```python
from build123d import *

# Parameters (mm, degrees)
F3_DEPTH = 10


with BuildPart() as f3:
    # F2 (on face) → F3 (new body)
    with BuildSketch(Plane.XY):
        with BuildLine():
            ThreePointArc((-207.1709679964, -147.5133103132), (-207.6520447758, -144.8452854186), (-209.0346813202, -142.5133103132))
            Line((-209.0346813202, -142.5133103132), (-209.0346813202, -152.5133103132))
            ThreePointArc((-209.0346813202, -152.5133103132), (-207.6520447758, -150.1813352079), (-207.1709679964, -147.5133103132))
        make_face()
        with BuildLine():
            Line((-139.082004335, -142.5133103132), (-209.0346813202, -142.5133103132))
            ThreePointArc((-209.0346813202, -142.5133103132), (-207.6520447758, -144.8452854186), (-207.1709679964, -147.5133103132))
            ThreePointArc((-207.1709679964, -147.5133103132), (-207.6520447758, -150.1813352079), (-209.0346813202, -152.5133103132))
            Line((-209.0346813202, -152.5133103132), (-139.082004335, -152.5133103132))
            ThreePointArc((-139.082004335, -152.5133103132), (-141.2519729984, -147.5133103132), (-139.082004335, -142.5133103132))
        make_face()
        with BuildLine():
            Line((-209.0346813202, -152.5133103132), (-209.0346813202, -142.5133103132))
            ThreePointArc((-209.0346813202, -142.5133103132), (-222.4487615225, -147.5133103132), (-209.0346813202, -152.5133103132))
        make_face()
        with BuildLine():
            ThreePointArc((-127.5611006367, -147.5133103132), (-131.6812494932, -141.2337557505), (-139.082004335, -142.5133103132))
            Line((-139.082004335, -142.5133103132), (-139.0346813202, -142.5133103132))
            Line((-139.0346813202, -142.5133103132), (-139.0346813202, -152.5133103132))
            Line((-139.0346813202, -152.5133103132), (-139.082004335, -152.5133103132))
            ThreePointArc((-139.082004335, -152.5133103132), (-131.6812494932, -153.792864876), (-127.5611006367, -147.5133103132))
        make_face()
        with BuildLine():
            Line((-139.0346813202, -142.5133103132), (-139.082004335, -142.5133103132))
            ThreePointArc((-139.082004335, -142.5133103132), (-141.2519729984, -147.5133103132), (-139.082004335, -152.5133103132))
            Line((-139.082004335, -152.5133103132), (-139.0346813202, -152.5133103132))
            Line((-139.0346813202, -152.5133103132), (-139.0346813202, -142.5133103132))
        make_face()
    extrude(amount=F3_DEPTH)


solid = f3.part
```
Check sheet for the modelled part. Datum: model origin and axes. Units: mm. A direction names the side the tool comes from. Round coordinates to 2 decimals unless told otherwise and drop trailing zeros. Loops run counter-clockwise (first coordinate to the right, second up) from the corner with the lowest first, then second, coordinate; pieces in that order, holes last. Notation, with made-up numbers: (-15.5, 68) - (23.5, 68) arc R24 cw to (23.5, 93) - close; hole circle Ø9 at (56.5, 59.5). An arc over 180 degrees is marked (long way). Answer as a JSON object with one key per item and string values. Group by question number.
Q1. Set-up check for faces 1 (the face through (-222.444, -147.254, 4.93)), 2 (the face through (-174, -142.513, 5)): record each of +Z, -Z, +X, -X, +Y, -Y from which the full face is reachable in a straight line by a thin tool's end or side.
Q2. Sectioned sample at B-B, the plane x = -173. Enter the section's corners in (y, z).
Q3. Gauge pin test, flat ends, axial feed: P1, Ø4, axis at y = -142.5, z = 6, coming from the +X side; P2, Ø4, axis at x = -149.5, y = -148, coming from the -Z side; P3, Ø5, axis at x = -173, z = 6.5, coming from the +Y side; P4, Ø3, axis at x = -182.5, z = 4.5, coming from the -Y side. Record the tip position at first contact, or that the pin passes through.
Q4. Scan lines: line 1 along Y through (x, z) = (-175, 1.5); line 2 along X through (y, z) = (-153.25, 1.75); line 3 along X through (y, z) = (-142, 1). Record each from-to range of solid material in increasing order. Write a range as [from, to].
Q5. Sectioned sample at C-C, the plane y = -143.5. Enter the section's corners in (x, z).
Q6. Sectioned sample at A-A, the plane z = 3. Enter the section's corners in (x, y).
Q7. Mould release check, pull along X, two halves, no side actions. Record for faces 3 (the face through (-176, -147, 10)), 4 (the face through (-175, -152.513, 5)): released by +X, released by -X, zero draft, split by the parting line, or undercut.
Solution:
{
 "1": {"face 1": "+Z, -Z", "face 2": "+Z, -Z, +Y"},
 "2": {"outline": "(-152.51, 0) - (-142.51, 0) - (-142.51, 10) - (-152.51, 10) - close"},
 "3": {"P1": "stops at x = -128.26", "P2": "stops at z = 0", "P3": "stops at y = -142.51", "P4": "stops at y = -152.51"},
 "4": {"line 1": "y = [-152.51, -142.51]", "line 2": "x = [-219.85, -209.77], [-138.14, -130.67]", "line 3": "x = [-220.1, -209.52], [-138.46, -130.35]"},
 "5": {"outline": "(-221.31, 0) - (-128.86, 0) - (-128.86, 10) - (-221.31, 10) - close"},
 "6": {"outline": "(-209.03, -152.51) - (-139.08, -152.51) arc R6.85 ccw (long way) to (-139.08, -142.51) - (-209.03, -142.51) arc R7.64 ccw (long way) to start"},
 "7": {"face 3": "zero draft", "face 4": "undercut"}
}
